Read the model definition and answer for the solid it produces. Units are mm, in the model's axes. Give positions to 0.01 mm unless a question says otherwise; leave off trailing zeros. Loops run counter-clockwise (first coordinate to the right, second up) from the corner with the lowest first, then second, coordinate; pieces in that order, holes last. Notation, with made-up numbers: (61, -17.5) -> (77, -17.5) arc R5 cw to (77, -9.5) -> close; hole circle Ø1 at (39, 37). An arc over 180 degrees is marked (long way). Return JSON: item names as keys, results as strings. Group by question number.
from build123d import *

# Parameters (mm, degrees)
SKETCH_1_W           = 250
SKETCH_1_H           = 150
EXTRUDE_1_DEPTH      = 5
SKETCH_1_4_R         = 3
CUT_EXTRUDE_1_DEPTH  = 5
SKETCH_1_5_R         = 3
CUT_EXTRUDE_2_DEPTH  = 5
SKETCH_1_6_R         = 3
CUT_EXTRUDE_3_DEPTH  = 5
SKETCH_1_7_R         = 3
CUT_EXTRUDE_4_DEPTH  = 5
SKETCH_2_R           = 3
CUT_EXTRUDE_5_DEPTH  = 5
SKETCH_3_R           = 3
CUT_EXTRUDE_6_DEPTH  = 45
SKETCH_3_3_R         = 3.5
CUT_EXTRUDE_7_DEPTH  = 45
SKETCH_4_R           = 3
CUT_EXTRUDE_8_DEPTH  = 5
SKETCH_4_3_R         = 3
CUT_EXTRUDE_9_DEPTH  = 5
SKETCH_5_R           = 3
CUT_EXTRUDE_10_DEPTH = 5
SKETCH_6_W           = 250
SKETCH_6_H           = 150
SKETCH_6_R           = 3
SKETCH_6_R_2         = 3.5
CUT_EXTRUDE_11_DEPTH = 1.5
SKETCH_7_R           = 3
CUT_EXTRUDE_12_DEPTH = 205.296965225
SKETCH_8_W           = 82.621849766
SKETCH_8_H           = 181.309059209
CUT_EXTRUDE_13_DEPTH = 10
CUT_EXTRUDE_14_DEPTH = 2


with BuildPart() as part:
    # Sketch 1 → Extrude 1 (new body)
    with BuildSketch(Plane(origin=(0, 0, 0), x_dir=(1, 0, 0), z_dir=(0, 1, 0))):
        with Locations((-65, 0)):
            Rectangle(SKETCH_1_W, SKETCH_1_H)
    extrude(amount=-EXTRUDE_1_DEPTH)

    # Sketch 1_4 → Cut-Extrude 1 (cut)
    with BuildSketch(Plane(origin=(0, 0, 0), x_dir=(1, 0, 0), z_dir=(0, 1, 0))):
        with Locations(Location((0, 50, 0), (0, 0, 270))):
            Circle(SKETCH_1_4_R)
    extrude(amount=-CUT_EXTRUDE_1_DEPTH, mode=Mode.SUBTRACT)

    # Sketch 1_5 → Cut-Extrude 2 (cut)
    with BuildSketch(Plane(origin=(0, 0, 0), x_dir=(1, 0, 0), z_dir=(0, 1, 0))):
        with Locations(Location((-50, 0, 0), (0, 0, 270))):
            Circle(SKETCH_1_5_R)
    extrude(amount=-CUT_EXTRUDE_2_DEPTH, mode=Mode.SUBTRACT)

    # Sketch 1_6 → Cut-Extrude 3 (cut)
    with BuildSketch(Plane(origin=(0, 0, 0), x_dir=(1, 0, 0), z_dir=(0, 1, 0))):
        with Locations(Location((0, -50, 0), (0, 0, 270))):
            Circle(SKETCH_1_6_R)
    extrude(amount=-CUT_EXTRUDE_3_DEPTH, mode=Mode.SUBTRACT)

    # Sketch 1_7 → Cut-Extrude 4 (cut)
    with BuildSketch(Plane(origin=(0, 0, 0), x_dir=(1, 0, 0), z_dir=(0, 1, 0))):
        with Locations(Location((50, 0, 0), (0, 0, 270))):
            Circle(SKETCH_1_7_R)
    extrude(amount=-CUT_EXTRUDE_4_DEPTH, mode=Mode.SUBTRACT)

    # Sketch 2 → Cut-Extrude 5 (cut)
    with BuildSketch(Plane(origin=(0, 0, 0), x_dir=(1, 0, 0), z_dir=(0, 1, 0))):
        with Locations(Location((-150.76, -37.46, 0), (0, 0, 270))):
            Circle(SKETCH_2_R)
    extrude(amount=-CUT_EXTRUDE_5_DEPTH, mode=Mode.SUBTRACT)

    # Sketch 3 → Cut-Extrude 6 (cut)
    with BuildSketch(Plane(origin=(0, 0, 0), x_dir=(1, 0, 0), z_dir=(0, 1, 0))):
        with Locations(Location((-132.57, -37.93, 0), (0, 0, 270))):
            Circle(SKETCH_3_R)
    extrude(amount=-CUT_EXTRUDE_6_DEPTH, mode=Mode.SUBTRACT)

    # Sketch 3_3 → Cut-Extrude 7 (cut)
    with BuildSketch(Plane(origin=(0, 0, 0), x_dir=(1, 0, 0), z_dir=(0, 1, 0))):
        with Locations(Location((-138.16, -24.34, 0), (0, 0, 270))):
            Circle(SKETCH_3_3_R)
    extrude(amount=-CUT_EXTRUDE_7_DEPTH, mode=Mode.SUBTRACT)

    # Sketch 4 → Cut-Extrude 8 (cut)
    with BuildSketch(Plane(origin=(0, 0, 0), x_dir=(1, 0, 0), z_dir=(0, 1, 0))):
        with Locations(Location((-112.5, -50, 0), (0, 0, 270))):
            Circle(SKETCH_4_R)
    extrude(amount=-CUT_EXTRUDE_8_DEPTH, mode=Mode.SUBTRACT)

    # Sketch 4_3 → Cut-Extrude 9 (cut)
    with BuildSketch(Plane(origin=(0, 0, 0), x_dir=(1, 0, 0), z_dir=(0, 1, 0))):
        with Locations(Location((-64.5, -50, 0), (0, 0, 270))):
            Circle(SKETCH_4_3_R)
    extrude(amount=-CUT_EXTRUDE_9_DEPTH, mode=Mode.SUBTRACT)

    # Sketch 5 → Cut-Extrude 10 (cut)
    with BuildSketch(Plane(origin=(0, 0, 0), x_dir=(1, 0, 0), z_dir=(0, 1, 0))):
        with Locations(Location((-112.61, -18.84, 0), (0, 0, 270))):
            Circle(SKETCH_5_R)
        with Locations(Location((-101.14, 21.42, 0), (0, 0, 270))):
            Circle(SKETCH_5_R)
    extrude(amount=-CUT_EXTRUDE_10_DEPTH, mode=Mode.SUBTRACT)

    # Sketch 6 → Cut-Extrude 11 (cut)
    with BuildSketch(Plane(origin=(0, 0, 0), x_dir=(1, 0, 0), z_dir=(0, 1, 0))):
        with Locations((-65, 0)):
            Rectangle(SKETCH_6_W, SKETCH_6_H)
        with Locations(Location((-150.76, -37.46, 0), (0, 0, 270))):
            Circle(SKETCH_6_R, mode=Mode.SUBTRACT)
        with Locations(Location((-138.16, -24.34, 0), (0, 0, 270))):
            Circle(SKETCH_6_R_2, mode=Mode.SUBTRACT)
        with Locations(Location((-132.57, -37.93, 0), (0, 0, 270))):
            Circle(SKETCH_6_R, mode=Mode.SUBTRACT)
        with Locations(Location((-112.61, -18.84, 0), (0, 0, 270))):
            Circle(SKETCH_6_R, mode=Mode.SUBTRACT)
        with Locations(Location((-112.5, -50, 0), (0, 0, 270))):
            Circle(SKETCH_6_R, mode=Mode.SUBTRACT)
        with Locations(Location((-101.14, 21.42, 0), (0, 0, 270))):
            Circle(SKETCH_6_R, mode=Mode.SUBTRACT)
        with Locations(Location((-50, 0, 0), (0, 0, 270))):
            Circle(SKETCH_6_R, mode=Mode.SUBTRACT)
        with Locations(Location((-64.5, -50, 0), (0, 0, 270))):
            Circle(SKETCH_6_R, mode=Mode.SUBTRACT)
        with Locations(Location((0, 50, 0), (0, 0, 270))):
            Circle(SKETCH_6_R, mode=Mode.SUBTRACT)
        with Locations(Location((0, -50, 0), (0, 0, 270))):
            Circle(SKETCH_6_R, mode=Mode.SUBTRACT)
        with Locations(Location((50, 0, 0), (0, 0, 270))):
            Circle(SKETCH_6_R, mode=Mode.SUBTRACT)
    extrude(amount=-CUT_EXTRUDE_11_DEPTH, mode=Mode.SUBTRACT)

    # Sketch 7 → Cut-Extrude 12 (cut, through all)
    with BuildSketch(Plane(origin=(0, -1.5, 0), x_dir=(1, 0, 0), z_dir=(0, 1, 0))):
        with Locations(Location((-64.5, 50, 0), (0, 0, 270))):
            Circle(SKETCH_7_R)
        with Locations(Location((-112.5, 50, 0), (0, 0, 270))):
            Circle(SKETCH_7_R)
        with Locations(Location((-64.5, -50, 0), (0, 0, 270))):
            Circle(SKETCH_7_R)
        with Locations(Location((-112.5, -50, 0), (0, 0, 270))):
            Circle(SKETCH_7_R)
    extrude(amount=-CUT_EXTRUDE_12_DEPTH, mode=Mode.SUBTRACT)

    # Sketch 8 → Cut-Extrude 13 (cut)
    with BuildSketch(Plane(origin=(0, -1.5, 0), x_dir=(1, 0, 0), z_dir=(0, 1, 0))):
        with Locations((-211.310924883, 0.092792435)):
            Rectangle(SKETCH_8_W, SKETCH_8_H)
    extrude(amount=-CUT_EXTRUDE_13_DEPTH, mode=Mode.SUBTRACT)

    # Sketch 11 → Cut-Extrude 14 (cut)
    with BuildSketch(Plane(origin=(0, -1.5, 0), x_dir=(1, 0, 0), z_dir=(0, 1, 0))):
        with BuildLine():
            Line((-165.849119967, -37.512806521), (-166.841935203, -37.632463975))
            ThreePointArc((-166.841935203, -37.632463975), (-159.595989048, -51.4607747), (-145, -57))
            Line((-145, -57), (-145, -56))
            ThreePointArc((-145, -56), (-158.932535, -50.712557668), (-165.849119967, -37.512806521))
        make_face()
    cut_extrude_14 = extrude(amount=-CUT_EXTRUDE_14_DEPTH, mode=Mode.SUBTRACT)

    # Mirror 1: Cut-Extrude 14 across plane
    add(cut_extrude_14.mirror(Plane.XY.offset(37.46)), mode=Mode.SUBTRACT)


solid = part.part
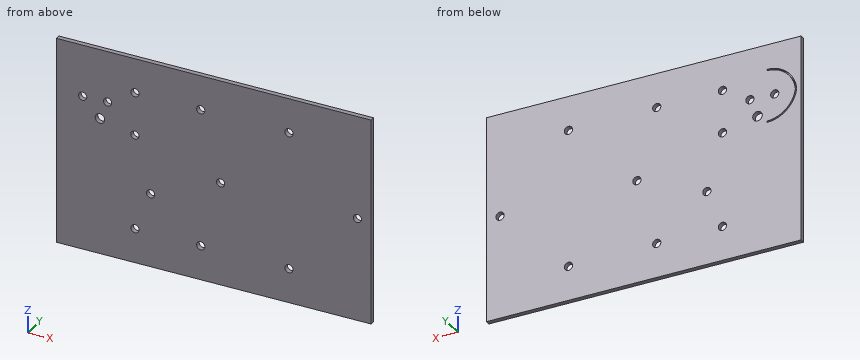
1. Straight lines are drawn through the part: line 1 (X direction, y = -4.2, z = 37.46); line 2 (X direction, y = -3.8, z = 0); line 3 (X direction, y = -2.45, z = -50). For each, find the intervals that lie inside material, in ascending order. Write a range as from..to.
2. Section C-C on z = -21.42 is taken. Determine the outline of the cut face in (x, y).
3. Section D-D on z = 0 is taken. Determine the outline of the cut face in (x, y).
4. A flat-ended cylindrical pin translates along its axis: pin 1 Ø5.5 at (x, z) = (-112.5, -50) entering from -Y. Find the tip coordinate at first contact, or state that the pin passes through.
5. Section A-A on z = -50 is taken. Determine the outline of the cut face in (x, y).
6. Section B-B on x = 50 is taken. Determine the outline of the cut face in (y, z).
Completed:
{
 "1": {"line 1": "x = -170..-153.76, -147.76..-135.53, -129.61..60", "line 2": "x = -170..-53, -47..47, 53..60", "line 3": "x = -170..-115.5, -109.5..-67.5, -61.5..-3, 3..60"},
 "2": {"outline": "(-170, -5) -> (-104.14, -5) -> (-104.14, -1.5) -> (-170, -1.5) -> close; (-98.14, -5) -> (60, -5) -> (60, -1.5) -> (-98.14, -1.5) -> close"},
 "3": {"outline": "(-170, -5) -> (-53, -5) -> (-53, -1.5) -> (-170, -1.5) -> close; (-47, -5) -> (47, -5) -> (47, -1.5) -> (-47, -1.5) -> close; (53, -5) -> (60, -5) -> (60, -1.5) -> (53, -1.5) -> close"},
 "4": {"pin 1": "passes through"},
 "5": {"outline": "(-170, -5) -> (-115.5, -5) -> (-115.5, -1.5) -> (-170, -1.5) -> close; (-109.5, -5) -> (-67.5, -5) -> (-67.5, -1.5) -> (-109.5, -1.5) -> close; (-61.5, -5) -> (-3, -5) -> (-3, -1.5) -> (-61.5, -1.5) -> close; (3, -5) -> (60, -5) -> (60, -1.5) -> (3, -1.5) -> close"},
 "6": {"outline": "(-5, -75) -> (-1.5, -75) -> (-1.5, -3) -> (-5, -3) -> close; (-5, 3) -> (-1.5, 3) -> (-1.5, 75) -> (-5, 75) -> close"}
}
